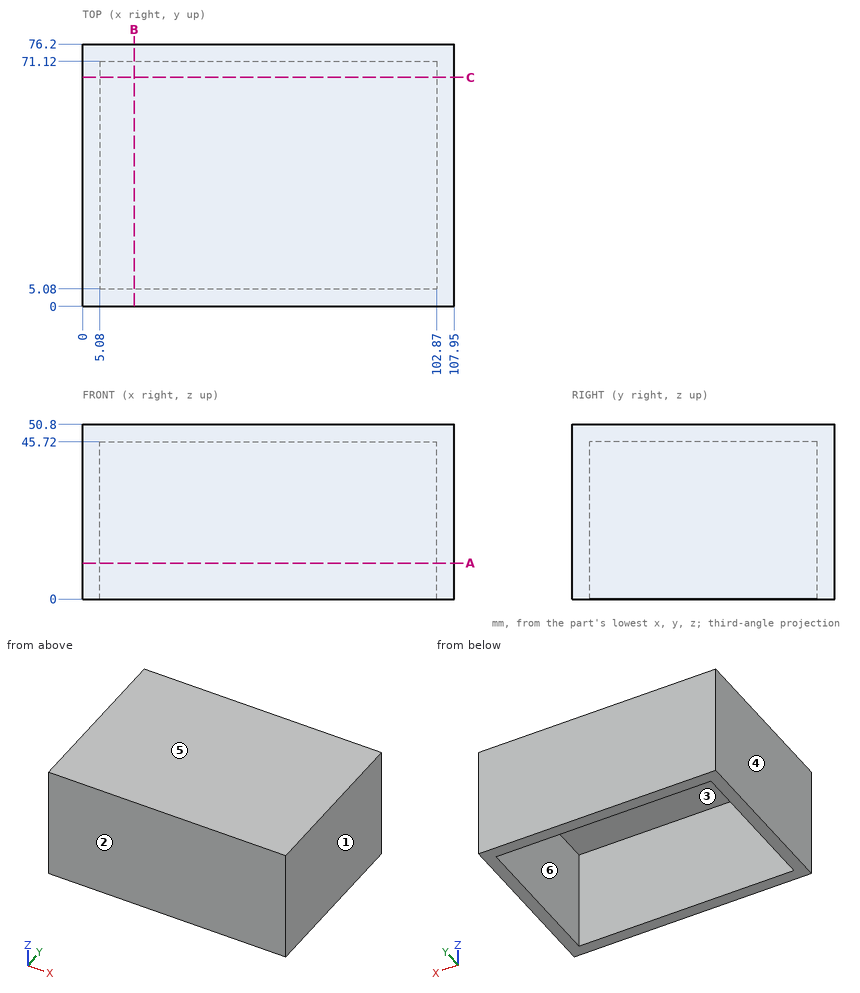
Can you work these out from the drawing? Everything is in mm from the part's minimum corner. A direction names the side the tool comes from. Round coordinates to 2 decimals unless told otherwise and drop trailing zeros. Write each loop counter-clockwise with the first axis right and the second up, starting at its lowest first coordinate (ties: lowest second). Pieces come first, ordered by that corner, then holes. Notation, with made-up numbers: (-25, 31) - (9, 31) arc R34 cw to (9, 67) - close; hole circle Ø1 at (-17, 43). An arc over 180 degrees is marked (long way). Put each result on its own line as item: value. Start each with the question number.
(1) I want a section at A-A, the plane z = 10.5. Please give me the cut outline in (x, y), plus the area to 3 significant figures.
(2) Thinking about a two-plate mould opening in X: for the marked faces 1, 2, 3 and 4, which applies, released by +X, released by -X, zero draft, split by the parting line, or undercut?
(3) Will these pins go through, and if not, where does the flat tip stop? pin 1 (10 mm diameter, centred on y = 36, z = 33.5, fed in from -X); pin 2 (10 mm diameter, centred on x = 39.5, y = 35, fed in from -Z).
(4) For the marked faces 5 and 6, which set-ups out of +Z, -Z, +X, -X, +Y, -Y let a thin tool reach every point of the face, with its end or its side?
(5) I want a section at B-B, the plane x = 15. Please give me the cut outline in (y, z).
(6) I want a section at C-C, the plane y = 66.5. Please give me the cut outline in (x, z).
(7) I need wall thicknesses on probe 1 along Y at (x, z) = (10, 28.5); probe 2 along X at (y, z) = (16.5, 20); probe 3 along Z at (x, y) = (91, 55.5). Which ranges of each line are inside material? Lowest first, please.
Here are the results:
1. outline: (0, 0) - (107.95, 0) - (107.95, 76.2) - (0, 76.2) - close; hole (5.08, 5.08) - (102.87, 5.08) - (102.87, 71.12) - (5.08, 71.12) - close
1. area: 1,770 mm^2
2. face 1: released by +X
2. face 2: zero draft
2. face 3: undercut
2. face 4: released by -X
3. pin 1: stops at x = 0
3. pin 2: stops at z = 45.72
4. face 5: +Z, +X, -X, +Y, -Y
4. face 6: -Z
5. outline: (0, 0) - (5.08, 0) - (5.08, 45.72) - (71.12, 45.72) - (71.12, 0) - (76.2, 0) - (76.2, 50.8) - (0, 50.8) - close
6. outline: (0, 0) - (5.08, 0) - (5.08, 45.72) - (102.87, 45.72) - (102.87, 0) - (107.95, 0) - (107.95, 50.8) - (0, 50.8) - close
7. probe 1: y = 0 to 5.08, 71.12 to 76.2
7. probe 2: x = 0 to 5.08, 102.87 to 107.95
7. probe 3: z = 45.72 to 50.8
